Can you work these out from the model? Positions are in its coordinate system, mm. Round coordinates to 2 decimals unless told otherwise and drop trailing zeros. Loops run counter-clockwise (first coordinate to the right, second up) from the corner with the lowest first, then second, coordinate; pieces in that order, holes last.
```python
from build123d import *

# Parameters (mm, degrees)
EXTRUDE_1_DEPTH   = 3
HOLE_WIZARD_M31_D = 3.15
CHAMFER_2_SIZE    = 0.25


with BuildPart() as part:
    # Эскиз1 → Бобышка-Вытянуть1 (new body)
    with BuildSketch(Plane.XY):
        with BuildLine():
            Line((-25.4, -48.25), (25.4, -48.25))
            ThreePointArc((25.4, -48.25), (28.652691193, -46.902691193), (30, -43.65))
            Line((30, -43.65), (30, 43.65))
            ThreePointArc((30, 43.65), (28.652691193, 46.902691193), (25.4, 48.25))
            Line((25.4, 48.25), (-25.4, 48.25))
            ThreePointArc((-25.4, 48.25), (-28.652691193, 46.902691193), (-30, 43.65))
            Line((-30, 43.65), (-30, -43.65))
            ThreePointArc((-30, -43.65), (-28.652691193, -46.902691193), (-25.4, -48.25))
        make_face()
        with BuildLine():
            Line((-12.55, -40.2), (-12.55, -18.7))
            ThreePointArc((-12.55, -18.7), (-10, -16.15), (-7.45, -18.7))
            Line((-7.45, -18.7), (-7.45, -40.2))
            ThreePointArc((-7.45, -40.2), (-10, -42.75), (-12.55, -40.2))
        make_face(mode=Mode.SUBTRACT)
        with BuildLine():
            Line((-22.55, -40.2), (-22.55, -18.7))
            ThreePointArc((-22.55, -18.7), (-20, -16.15), (-17.45, -18.7))
            Line((-17.45, -18.7), (-17.45, -40.2))
            ThreePointArc((-17.45, -40.2), (-20, -42.75), (-22.55, -40.2))
        make_face(mode=Mode.SUBTRACT)
        with BuildLine():
            Line((-2.55, -40.2), (-2.55, -18.7))
            ThreePointArc((-2.55, -18.7), (0, -16.15), (2.55, -18.7))
            Line((2.55, -18.7), (2.55, -40.2))
            ThreePointArc((2.55, -40.2), (0, -42.75), (-2.55, -40.2))
        make_face(mode=Mode.SUBTRACT)
        with BuildLine():
            Line((7.45, -40.2), (7.45, -18.7))
            ThreePointArc((7.45, -18.7), (10, -16.15), (12.55, -18.7))
            Line((12.55, -18.7), (12.55, -40.2))
            ThreePointArc((12.55, -40.2), (10, -42.75), (7.45, -40.2))
        make_face(mode=Mode.SUBTRACT)
        with BuildLine():
            Line((17.45, -40.2), (17.45, -18.7))
            ThreePointArc((17.45, -18.7), (20, -16.15), (22.55, -18.7))
            Line((22.55, -18.7), (22.55, -40.2))
            ThreePointArc((22.55, -40.2), (20, -42.75), (17.45, -40.2))
        make_face(mode=Mode.SUBTRACT)
        with BuildLine():
            Line((-16.62137085, 32.90862915), (-14.589639684, 30.876897984))
            ThreePointArc((-14.589639684, 30.876897984), (-19.1, 18.55), (-14.589639684, 6.223102016))
            Line((-14.589639684, 6.223102016), (-16.62137085, 4.19137085))
            ThreePointArc((-16.62137085, 4.19137085), (-16.62137085, 1.92862915), (-14.35862915, 1.92862915))
            Line((-14.35862915, 1.92862915), (-12.326897984, 3.960360316))
            ThreePointArc((-12.326897984, 3.960360316), (0, -0.55), (12.326897984, 3.960360316))
            Line((12.326897984, 3.960360316), (14.35862915, 1.92862915))
            ThreePointArc((14.35862915, 1.92862915), (16.62137085, 1.92862915), (16.62137085, 4.19137085))
            Line((16.62137085, 4.19137085), (14.589639684, 6.223102016))
            ThreePointArc((14.589639684, 6.223102016), (19.1, 18.55), (14.589639684, 30.876897984))
            Line((14.589639684, 30.876897984), (16.62137085, 32.90862915))
            ThreePointArc((16.62137085, 32.90862915), (16.62137085, 35.17137085), (14.35862915, 35.17137085))
            Line((14.35862915, 35.17137085), (12.326897984, 33.139639684))
            ThreePointArc((12.326897984, 33.139639684), (0, 37.65), (-12.326897984, 33.139639684))
            Line((-12.326897984, 33.139639684), (-14.35862915, 35.17137085))
            ThreePointArc((-14.35862915, 35.17137085), (-16.62137085, 35.17137085), (-16.62137085, 32.90862915))
        make_face(mode=Mode.SUBTRACT)
    extrude(amount=EXTRUDE_1_DEPTH)

    # Сверло под метчик  спиральное M31 (through all)
    with Locations(Plane.XY.offset(3)):
        with Locations((-23.55, 42.1), (23.55, 42.1), (23.55, -5), (-23.55, -5)):
            Hole(HOLE_WIZARD_M31_D / 2)

    # Фаска2
    chamfer_2_edges = [part.edges().sort_by_distance(p)[0] for p in [
        (28.652691193, -46.902691193, 3),
        (0, -48.25, 0),
        (-28.652691193, -46.902691193, 0),
        (10, -16.15, 0),
        (7.45, -29.45, 0),
        (10, -42.75, 0),
        (12.55, -29.45, 0),
        (10, -16.15, 3),
        (7.45, -29.45, 3),
        (10, -42.75, 3),
        (12.55, -29.45, 3),
        (20, -16.15, 0),
        (17.45, -29.45, 0),
        (20, -42.75, 0),
        (22.55, -29.45, 0),
        (20, -16.15, 3),
        (17.45, -29.45, 3),
        (20, -42.75, 3),
        (22.55, -29.45, 3),
        (30, 0, 3),
        (-21.975, -5, 3),
        (-21.975, -5, 0),
        (25.125, -5, 3),
        (25.125, -5, 0),
        (25.125, 42.1, 3),
        (25.125, 42.1, 0),
        (28.652691193, 46.902691193, 3),
        (-21.975, 42.1, 3),
        (-21.975, 42.1, 0),
        (0, 48.25, 3),
        (-28.652691193, 46.902691193, 3),
        (-30, 0, 3),
        (19.1, 18.55, 0),
        (15.605505267, 31.892763567, 0),
        (16.62137085, 35.17137085, 0),
        (13.342763567, 34.155505267, 0),
        (0, 37.65, 0),
        (-13.342763567, 34.155505267, 0),
        (-16.62137085, 35.17137085, 0),
        (-15.605505267, 31.892763567, 0),
        (-19.1, 18.55, 0),
        (-15.605505267, 5.207236433, 0),
        (-16.62137085, 1.92862915, 0),
        (-13.342763567, 2.944494733, 0),
        (0, -0.55, 0),
        (13.342763567, 2.944494733, 0),
        (16.62137085, 1.92862915, 0),
        (15.605505267, 5.207236433, 0),
        (19.1, 18.55, 3),
        (15.605505267, 31.892763567, 3),
        (-28.652691193, -46.902691193, 3),
        (16.62137085, 35.17137085, 3),
        (13.342763567, 34.155505267, 3),
        (0, 37.65, 3),
        (-13.342763567, 34.155505267, 3),
        (-16.62137085, 35.17137085, 3),
        (-15.605505267, 31.892763567, 3),
        (-19.1, 18.55, 3),
        (-15.605505267, 5.207236433, 3),
        (-16.62137085, 1.92862915, 3),
        (-13.342763567, 2.944494733, 3),
        (0, -0.55, 3),
        (13.342763567, 2.944494733, 3),
        (16.62137085, 1.92862915, 3),
        (15.605505267, 5.207236433, 3),
        (-20, -16.15, 0),
        (-22.55, -29.45, 0),
        (-20, -42.75, 0),
        (0, -48.25, 3),
        (-17.45, -29.45, 0),
        (-20, -16.15, 3),
        (-22.55, -29.45, 3),
        (-20, -42.75, 3),
        (-17.45, -29.45, 3),
        (-30, 0, 0),
        (-28.652691193, 46.902691193, 0),
        (-10, -16.15, 0),
        (-12.55, -29.45, 0),
        (-10, -42.75, 0),
        (-7.45, -29.45, 0),
        (-10, -16.15, 3),
        (-12.55, -29.45, 3),
        (-10, -42.75, 3),
        (-7.45, -29.45, 3),
        (0, 48.25, 0),
        (28.652691193, 46.902691193, 0),
        (30, 0, 0),
        (0, -16.15, 0),
        (-2.55, -29.45, 0),
        (0, -42.75, 0),
        (2.55, -29.45, 0),
        (0, -16.15, 3),
        (-2.55, -29.45, 3),
        (28.652691193, -46.902691193, 0),
        (0, -42.75, 3),
        (2.55, -29.45, 3),
    ]]
    chamfer(chamfer_2_edges, length=CHAMFER_2_SIZE)


solid = part.part
```
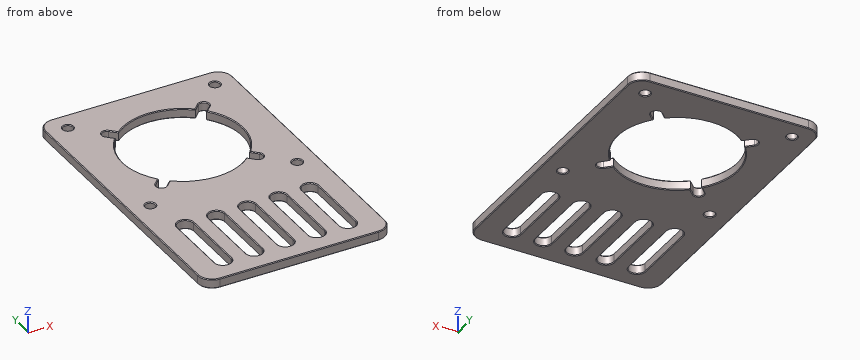
(1) Suppose I cut it at A-A (y = 42.1). Write out the boundary of the cut face in (x, z) (3 decimals).
(2) Suppose I cut it at B-B (z = 2.1). Give the number of separate pieces and of enclosed holes in the cut face, then the cut area to 3 significant figures.
(3) If I drill on line 1 (X direction, y = -30, z = 2.75); line 2 (Y direction, x = 23.55, z = 1) (3 decimals), over which ranges is the centre line in solid material (lowest first)?
Check result:
1. outline: (-30, 0.25) - (-29.75, 0) - (-25.375, 0) - (-25.125, 0.25) - (-25.125, 2.75) - (-25.375, 3) - (-29.75, 3) - (-30, 2.75) - close; (-21.975, 0.25) - (-21.725, 0) - (21.725, 0) - (21.975, 0.25) - (21.975, 2.75) - (21.725, 3) - (-21.725, 3) - (-21.975, 2.75) - close; (25.125, 0.25) - (25.375, 0) - (29.75, 0) - (30, 0.25) - (30, 2.75) - (29.75, 3) - (25.375, 3) - (25.125, 2.75) - close
2. separate pieces: 1
2. enclosed holes: 10
2. area: 3,890 mm2
3. line 1: x = -30 to -22.55, -17.45 to -12.55, -7.45 to -2.55, 2.55 to 7.45, 12.55 to 17.45, 22.55 to 30
3. line 2: y = -48.25 to -6.575, -3.425 to 40.525, 43.675 to 48.25
